```python
from build123d import *

# Parameters (mm, degrees)
F0_W     = 361.95
F0_H     = 692.15
F1_DEPTH = 581.025
F2_W     = 330.2
F2_H     = 660.4
F3_DEPTH = 565.15
F5_DEPTH = 565.15
F7_DEPTH = 25.4


# Not quite as in the source:
# - a feature names something its author has since deleted; it is built from what else it names


with BuildPart() as f1:
    # F0 (on Front) → F1 (new body)
    with BuildSketch(Plane.XZ):
        with Locations((180.975, 346.075)):
            Rectangle(F0_W, F0_H)
    extrude(amount=F1_DEPTH)

    # F2 (on face) → F3 (cut)
    with BuildSketch(Plane.XZ.offset(581.025)):
        with Locations((180.975, 346.075)):
            Rectangle(F2_W, F2_H)
    extrude(amount=-F3_DEPTH, mode=Mode.SUBTRACT)

    # F4 (on face) → F5 (join)
    with BuildSketch(Plane.XZ.offset(581.025)):
        Polygon((104.775, 168.275), (15.875, 168.275), (15.875, 15.875), (346.075, 15.875), (346.075, 168.275), (257.175, 168.275), (225.425, 149.225), (136.525, 149.225), align=None)
        Polygon((104.775, 676.275), (15.875, 676.275), (15.875, 574.675), (104.775, 574.675), (257.175, 574.675), (346.075, 574.675), (346.075, 676.275), (257.175, 676.275), (225.425, 657.225), (136.525, 657.225), align=None)
        Polygon((104.775, 574.675), (15.875, 574.675), (15.875, 473.075), (104.775, 473.075), (257.175, 473.075), (346.075, 473.075), (346.075, 574.675), (257.175, 574.675), (225.425, 555.625), (136.525, 555.625), align=None)
        Polygon((104.775, 473.075), (15.875, 473.075), (15.875, 320.675), (104.775, 320.675), (257.175, 320.675), (346.075, 320.675), (346.075, 473.075), (257.175, 473.075), (225.425, 454.025), (136.525, 454.025), align=None)
        Polygon((104.775, 320.675), (15.875, 320.675), (15.875, 168.275), (104.775, 168.275), (257.175, 168.275), (346.075, 168.275), (346.075, 320.675), (257.175, 320.675), (225.425, 301.625), (136.525, 301.625), align=None)
    extrude(amount=-F5_DEPTH)

    # F6 (on face) → F7 (cut)
    with BuildSketch(Plane.XZ.offset(581.025)):
        Polygon((257.175, 676.275), (104.775, 676.275), (109.0083333333, 673.735), (252.9416666667, 673.735), align=None)
        Polygon((104.775, 676.275), (15.875, 676.275), (15.875, 15.875), (346.075, 15.875), (346.075, 676.275), (257.175, 676.275), (252.9416666667, 673.735), (343.535, 673.735), (343.535, 574.675), (343.535, 572.135), (343.535, 473.075), (343.535, 470.535), (343.535, 320.675), (343.535, 318.135), (343.535, 168.275), (343.535, 165.735), (343.535, 18.415), (18.415, 18.415), (18.415, 165.735), (18.415, 168.275), (18.415, 318.135), (18.415, 320.675), (18.415, 470.535), (18.415, 473.075), (18.415, 572.135), (18.415, 574.675), (18.415, 673.735), (109.0083333333, 673.735), align=None)
        Polygon((257.175, 574.675), (104.775, 574.675), (109.0083333333, 572.135), (252.9416666667, 572.135), align=None)
        Polygon((104.775, 574.675), (18.415, 574.675), (18.415, 572.135), (109.0083333333, 572.135), align=None)
        Polygon((343.535, 572.135), (343.535, 574.675), (257.175, 574.675), (252.9416666667, 572.135), align=None)
        Polygon((343.535, 470.535), (343.535, 473.075), (257.175, 473.075), (252.9416666667, 470.535), align=None)
        Polygon((257.175, 473.075), (104.775, 473.075), (109.0083333333, 470.535), (252.9416666667, 470.535), align=None)
        Polygon((104.775, 473.075), (18.415, 473.075), (18.415, 470.535), (109.0083333333, 470.535), align=None)
        Polygon((257.175, 320.675), (104.775, 320.675), (109.0083333333, 318.135), (252.9416666667, 318.135), align=None)
        Polygon((104.775, 320.675), (18.415, 320.675), (18.415, 318.135), (109.0083333333, 318.135), align=None)
        Polygon((343.535, 318.135), (343.535, 320.675), (257.175, 320.675), (252.9416666667, 318.135), align=None)
        Polygon((343.535, 165.735), (343.535, 168.275), (257.175, 168.275), (252.9416666667, 165.735), align=None)
        Polygon((108.4452420473, 168.275), (104.775, 168.275), (109.0083333333, 165.735), (252.9416666667, 165.735), (257.175, 168.275), align=None)
        Polygon((104.775, 168.275), (18.415, 168.275), (18.415, 165.735), (109.0083333333, 165.735), align=None)
    extrude(amount=-F7_DEPTH, mode=Mode.SUBTRACT)


solid = f1.part
```
Could you check a few things on this model? Use its own coordinates, in mm. A direction names the side the tool comes from. Coordinates: 2 decimals unless noted, no trailing zeros. Loops run counter-clockwise (first coordinate to the right, second up) from the corner with the lowest first, then second, coordinate; pieces in that order, holes last.
1) Imagine slicing it at A-A (y = -136). List the corners of the cut face in (x, z) for me (3 decimals), and give its area (3 significant figures).
Reported:
outline: (0, 0) - (361.95, 0) - (361.95, 692.15) - (0, 692.15) - close; hole (104.775, 168.275) - (136.525, 149.225) - (225.425, 149.225) - (257.175, 168.275) - close; hole (104.775, 320.675) - (136.525, 301.625) - (225.425, 301.625) - (257.175, 320.675) - close; hole (104.775, 473.075) - (136.525, 454.025) - (225.425, 454.025) - (257.175, 473.075) - close; hole (104.775, 574.675) - (136.525, 555.625) - (225.425, 555.625) - (257.175, 574.675) - close; hole (104.775, 676.275) - (136.525, 657.225) - (225.425, 657.225) - (257.175, 676.275) - close
area: 239,000 mm2
2) Thinking about a two-plate mould opening in X: for faces 3 (the face through (182, -302, 555.625)), 4 (the face through (179, -581.025, 523)), 5 (the face through (0, -286, 341)), which applies, released by +X, released by -X, zero draft, split by the parting line, or undercut?
Reported:
face 3: undercut
face 4: zero draft
face 5: released by -X
3) Please list where these lines run through material, in increasing order: line 1 along Z through (x, y) = (156, -322) (3 decimals); line 2 along Z through (x, y) = (256, -137.5) (3 decimals); line 3 along Y through (x, z) = (345, 192.5) (3 decimals).
Reported:
line 1: z = 0 to 149.225, 168.275 to 301.625, 320.675 to 454.025, 473.075 to 555.625, 574.675 to 657.225, 676.275 to 692.15
line 2: z = 0 to 167.57, 168.275 to 319.97, 320.675 to 472.37, 473.075 to 573.97, 574.675 to 675.57, 676.275 to 692.15
line 3: y = -555.625 to 0
4) Imagine slicing it at B-B (x = 185.5). List the corners of the cut face in (y, z) for me (3 decimals).
Reported:
outline: (-581.025, 0) - (0, 0) - (0, 692.15) - (-581.025, 692.15) - (-581.025, 676.275) - (-15.875, 676.275) - (-15.875, 657.225) - (-581.025, 657.225) - (-581.025, 574.675) - (-15.875, 574.675) - (-15.875, 555.625) - (-581.025, 555.625) - (-581.025, 473.075) - (-15.875, 473.075) - (-15.875, 454.025) - (-581.025, 454.025) - (-581.025, 320.675) - (-15.875, 320.675) - (-15.875, 301.625) - (-581.025, 301.625) - (-581.025, 168.275) - (-15.875, 168.275) - (-15.875, 149.225) - (-581.025, 149.225) - (-581.025, 18.415) - (-555.625, 18.415) - (-555.625, 15.875) - (-581.025, 15.875) - close
5) Which directions (+Z, -Z, +X, -X, +Y, -Y) give clear straight access to the entire face, cutting with the end or side of a thin tool? Please do faces 1 (the face through (361.95, -286, 341)), 2 (the face through (182, -302, 149.225)).
Reported:
face 1: +Z, -Z, +X, +Y, -Y
face 2: -Y
6) Imagine slicing it at C-C (z = 564). List the corners of the cut face in (x, y) for me (3 decimals).
Reported:
outline: (0, -581.025) - (15.875, -581.025) - (15.875, -555.625) - (18.415, -555.625) - (18.415, -581.025) - (122.567, -581.025) - (122.567, -15.875) - (239.383, -15.875) - (239.383, -581.025) - (343.535, -581.025) - (343.535, -555.625) - (346.075, -555.625) - (346.075, -581.025) - (361.95, -581.025) - (361.95, 0) - (0, 0) - close
